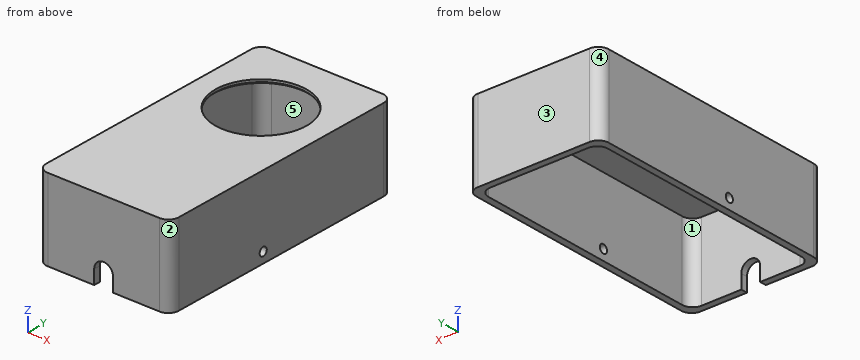
from build123d import *

# Parameters (mm, degrees)
SKETCH013_R             = 13
PAD007_DEPTH            = 23.2
POCKET006_DEPTH         = 22
CHAMFER_SIZE            = 0.5
POCKET017_DEPTH         = 5
SKETCH055_R             = 1.2
POCKET020012_DEPTH      = 38.001
BODY002_PLACEMENT_ANGLE = 180


with BuildPart() as part:
    # Sketch013 → Pad007 (new body)
    with BuildSketch(Plane.XY):
        with BuildLine():
            ThreePointArc((-48, 75), (-50.12132, 74.12132), (-51, 72))
            Line((-51, 3), (-51, 72))
            ThreePointArc((-51, 3), (-50.12132, 0.87868), (-48, 0))
            Line((-16, 0), (-48, 0))
            ThreePointArc((-16, 0), (-13.87868, 0.87868), (-13, 3))
            Line((-13, 72), (-13, 3))
            ThreePointArc((-13, 72), (-13.87868, 74.12132), (-16, 75))
            Line((-48, 75), (-16, 75))
        make_face()
        with Locations((-32, 53)):
            Circle(SKETCH013_R, mode=Mode.SUBTRACT)
    extrude(amount=PAD007_DEPTH)

    # Sketch014 (on Face11 of Pad007) → Pocket006 (cut)
    with BuildSketch(Plane.XY.offset(23.2)):
        with BuildLine():
            Line((-46.1, 73.1), (-17.9, 73.1))
            ThreePointArc((-14.9, 70.1), (-15.77868, 72.22132), (-17.9, 73.1))
            Line((-14.9, 70.1), (-14.9, 4.9))
            ThreePointArc((-17.9, 1.9), (-15.77868, 2.77868), (-14.9, 4.9))
            Line((-17.9, 1.9), (-46.1, 1.9))
            ThreePointArc((-49.1, 4.9), (-48.22132, 2.77868), (-46.1, 1.9))
            Line((-49.1, 4.9), (-49.1, 70.1))
            ThreePointArc((-46.1, 73.1), (-48.22132, 72.22132), (-49.1, 70.1))
        make_face()
    extrude(amount=-POCKET006_DEPTH, mode=Mode.SUBTRACT)

    # Chamfer
    chamfer_edges = [part.edges().sort_by_distance(p)[0] for p in [
        (-45, 53, 1.2),
    ]]
    chamfer(chamfer_edges, length=CHAMFER_SIZE)

    # Sketch031 → Pocket017 (cut)
    with BuildSketch(Plane.XZ):
        with BuildLine():
            ThreePointArc((-29.3, 25.058865), (-32, 27.758865), (-34.7, 25.058865))
            Line((-34.7, 25.058865), (-34.7, 19.2))
            ThreePointArc((-34.7, 19.2), (-32, 16.5), (-29.3, 19.2))
            Line((-29.3, 19.2), (-29.3, 25.058865))
        make_face()
    extrude(amount=-POCKET017_DEPTH, mode=Mode.SUBTRACT)

    # Sketch055 (on Face6 of Pocket017) → Pocket020012 (cut, through all)
    with BuildSketch(Plane(origin=(-51, 0, 0), x_dir=(0, -1, 0), z_dir=(-1, 0, 0))):
        with Locations((-31.42, 20.2)):
            Circle(SKETCH055_R)
    extrude(amount=-POCKET020012_DEPTH, mode=Mode.SUBTRACT)


with BuildPart() as part_1:
    # Body002 placement: moved
    add(part.part.moved(Location((-64, 0, 0))).rotate(Axis((-64, 0, 0), (0, 1, 0)), BODY002_PLACEMENT_ANGLE))


solid = part_1.part
The model under review builds one solid part; all positions refer to its coordinate system, in mm. Face numbers are marked on the shaded views. A direction names the side the tool comes from. Round coordinates to 2 decimals unless told otherwise and drop trailing zeros. Order: outer loops, then holes, each group sorted by start corner. A loop starts at its lowest first (then second) coordinate and runs counter-clockwise, first axis right, second up. Notation, with made-up numbers: (56, -23) - (73, -23) arc R17 cw to (73, 4) - close; hole circle Ø8 at (19, -17.5). An arc over 180 degrees is marked (long way). Use one line per item in the form item = value.
Q1. Add section A-A on x = -32. Give the boundary of the cut face in (y, z).
Response values:
outline = (0, -16.5) - (1.9, -16.5) - (1.9, -1.2) - (39.5, -1.2) - (40, -0.7) - (40, 0) - (0, 0) - close; (66, -0.7) - (66.5, -1.2) - (73.1, -1.2) - (73.1, -23.2) - (75, -23.2) - (75, 0) - (66, 0) - close
Q2. Clearance check with flat-ended pins moving along their axes: P1, Ø10, axis at x = -30, z = -20.5, coming from the -Y side; P2, Ø10.5, axis at x = -26.5, y = 53.5, coming from the -Z side; P3, Ø1, axis at y = 1, z = -22, coming from the -X side; P4, Ø1.5, axis at x = -45, y = 9, coming from the -Z side. State where each tip first meets the part, or that it passes through.
Response values:
P1 = 0
P2 = through
P3 = -50.6
P4 = -1.2
Q3. To check wall thickness, follow line 1 (X direction, y = 12.5, z = -4.5); line 2 (Y direction, x = -27, z = -2); line 3 (X direction, y = 53, z = -0.25). State the ranges of each line that lie inside material, in increasing order.
Response values:
line_1 = -51 to -49.1, -14.9 to -13
line_2 = 0 to 1.9, 73.1 to 75
line_3 = -51 to -45, -19 to -13
Q4. Add section B-B on y = 31.42. Give the boundary of the cut face in (x, z).
Response values:
outline = (-51, -23.2) - (-49.1, -23.2) - (-49.1, -21.4) - (-51, -21.4) - close; (-51, -19) - (-49.1, -19) - (-49.1, -1.2) - (-14.9, -1.2) - (-14.9, -19) - (-13, -19) - (-13, 0) - (-51, 0) - close; (-14.9, -23.2) - (-13, -23.2) - (-13, -21.4) - (-14.9, -21.4) - close
Q5. Mouldability with a two-part tool opening along X and no side actions: class the marked faces 1, 2 and 3 as pulls with the +X half, pulls with the -X half, needs draft (parallel to the pull), parting line crosses it, or undercut.
Response values:
face_1 = undercut
face_2 = pulls with the +X half
face_3 = needs draft
Q6. Tool access review of the marked faces 4 and 5: name each direction out of +Z, -Z, +X, -X, +Y, -Y from which nothing blocks a thin tool from reaching the whole face with its end or side.
Response values:
face_4 = +Z, -Z, -X, +Y
face_5 = -Z
Q7. Add section C-C on z = -6.75. Give the boundary of the cut face in (x, y), then the cut area to 3 significant figures.
Response values:
outline = (-51, 3) arc R3 ccw to (-48, 0) - (-16, 0) arc R3 ccw to (-13, 3) - (-13, 72) arc R3 ccw to (-16, 75) - (-48, 75) arc R3 ccw to (-51, 72) - close; hole (-49.1, 4.9) arc R3 ccw to (-46.1, 1.9) - (-17.9, 1.9) arc R3 ccw to (-14.9, 4.9) - (-14.9, 70.1) arc R3 ccw to (-17.9, 73.1) - (-46.1, 73.1) arc R3 ccw to (-49.1, 70.1) - close
area = 415 mm^2
Q8. Add section D-D on y = 53. Give the boundary of the cut face in (x, z).
Response values:
outline = (-51, -23.2) - (-49.1, -23.2) - (-49.1, -1.2) - (-45.5, -1.2) - (-45, -0.7) - (-45, 0) - (-51, 0) - close; (-19, -0.7) - (-18.5, -1.2) - (-14.9, -1.2) - (-14.9, -23.2) - (-13, -23.2) - (-13, 0) - (-19, 0) - close
